from build123d import *

# Parameters (mm, degrees)
F1_DEPTH = 454.025
F3_W     = 22.225
F3_H     = 3.96875
F4_DEPTH = 25.4
F5_W     = 13.49375
F5_H     = 3.96875
F6_DEPTH = 25.4


with BuildPart() as f1:
    # F0 (on Front) → F1 (new body)
    with BuildSketch(Plane.XZ):
        Polygon((-18.553972, 20.450408), (-21.728972, 20.450408), (-21.728972, -17.649592), (16.371028, -17.649592), (16.371028, -14.474592), (-18.553972, -14.474592), align=None)
    extrude(amount=F1_DEPTH)

    # F3 (on face) → F4 (cut)
    with BuildSketch(Plane(origin=(-21.728972, 0, 0), x_dir=(0, -1, 0), z_dir=(-1, 0, 0))):
        with Locations((442.9125, 18.466033)):
            Rectangle(F3_W, F3_H)
    extrude(amount=-F4_DEPTH, mode=Mode.SUBTRACT)

    # F5 (on face) → F6 (cut)
    with BuildSketch(Plane.XY.offset(-14.474592)):
        with Locations((9.624153, -102.790625)):
            Rectangle(F5_W, F5_H)
    extrude(amount=-F6_DEPTH, mode=Mode.SUBTRACT)


solid = f1.part
Input: part model. Units: mm. Frame: model coordinates. A direction names the side the tool comes from. Coordinates: 2 decimals unless noted, no trailing zeros. Loops run counter-clockwise (first coordinate to the right, second up) from the corner with the lowest first, then second, coordinate; pieces in that order, holes last.
(1) Set-up query: faces 1 (the face through (-11, -454.025, -16)), 2 (the face through (-18.554, -224, 3)). Return all of +Z, -Z, +X, -X, +Y, -Y with unobstructed straight access to the full face (end or side cutting, diameter ignored); none if empty.
(2) Material intervals for probe 1 along Z at (x, y) = (-3.5, -367); probe 2 along X at (y, z) = (-253.5, 6.5), sorted ascending.
(3) First-contact query: pin 1 Ø3.5 at (y, z) = (-102, -15.5) entering from +X; pin 2 Ø10.5 at (y, z) = (-267, 7.5) entering from +X; pin 3 Ø17.5 at (x, y) = (-5, -233) entering from +Z; pin 4 Ø3.5 at (x, z) = (-19.5, 19.5) entering from -Y. Flat tips, straight axial feed; report the tip coordinate or a pass-through.
(4) Section A-A on x = 8. Return the cut outline in (y, z) (3 decimals), then the cut area to 3 significant figures.
(5) Section B-B on z = 0. Return the cut outline in (x, y) (3 decimals).
(6) Section D-D on x = -10.5. Return the cut outline in (y, z) (3 decimals), then the cut area to 3 significant figures.
(7) Section C-C on y = -409. Return the cut outline in (x, z).
Data:
1. face 1: +Z, -Z, +X, -X, -Y
1. face 2: +Z, +X, +Y, -Y
2. probe 1: z = -17.65 to -14.47
2. probe 2: x = -21.73 to -18.55
3. pin 1: stops at x = 16.37
3. pin 2: stops at x = -18.55
3. pin 3: stops at z = -14.47
3. pin 4: stops at y = -431.8
4. outline: (-454.025, -17.65) - (-104.775, -17.65) - (-104.775, -14.475) - (-454.025, -14.475) - close; (-100.806, -17.65) - (0, -17.65) - (0, -14.475) - (-100.806, -14.475) - close
4. area: 1,430 mm2
5. outline: (-21.729, -454.025) - (-18.554, -454.025) - (-18.554, 0) - (-21.729, 0) - close
6. outline: (-454.025, -17.65) - (0, -17.65) - (0, -14.475) - (-454.025, -14.475) - close
6. area: 1,440 mm2
7. outline: (-21.73, -17.65) - (16.37, -17.65) - (16.37, -14.47) - (-18.55, -14.47) - (-18.55, 20.45) - (-21.73, 20.45) - close
